Here's how the part is built. I have some questions about the finished solid (model axes, mm). A direction names the side the tool comes from. Coordinates: 2 decimals unless noted, no trailing zeros. Write each loop counter-clockwise with the first axis right and the second up, starting at its lowest first coordinate (ties: lowest second). Pieces come first, ordered by that corner, then holes.
Item 1: If I drill on line 1 (X direction, y = -0.5, z = 1.1); line 2 (Y direction, x = -34, z = 3.8); line 3 (X direction, y = -5.25, z = 1.55), over which ranges is the centre line in solid material (lowest first)?
Item 2: We'd pull the mould along X, two halves only. Please class faces 1 (the face through (1, 0, 0)), 2 (the face through (54.15, -0.27, 2.96)), 3 (the face through (-12.918, -2.873, 2.958)), 4 (the face through (15.819, 3.575, 2.958)): +X half, -X half, draft (parallel to the pull), parting line (faces both ways), or undercut.
Item 3: For faces 5 (the face through (-34.37, -5.53, 4.52)), 6 (the face through (-31, -10, 3)), 7 (the face through (-42.6, -7.3, 3)), which set-ups out of +Z, -Z, +X, -X, +Y, -Y let a thin tool reach every point of the face, with its end or its side?
Item 4: If we section it at A-A (x = 8.5): Please give me the cut outline in (y, z), then the cut area to 3 significant figures.
Item 5: If we section it at C-C (x = -6): Please give me the cut outline in (y, z).
Item 6: If we section it at B-B (z = 1.3): Count the separate pieces of the cut face and the enclosed holes in it, then the cut area to 3 significant figures.
Item 7: I'm going to push flat-ended pins straight in: pin 1 Ø1 at (y, z) = (8.5, 4) entering from -X; pin 2 Ø1.5 at (y, z) = (-8, 4.5) entering from -X; pin 3 Ø3 at (y, z) = (-6.5, 4.5) entering from +X. Where does each tip first touch, or does it pass through?
Item 8: If we section it at D-D (x = -29): Please give me the cut outline in (y, z), then the cut area to 3 significant figures.
from build123d import *

# Parameters (mm, degrees)
SKETCH1_R                                       = 4
SKETCH1_R_2                                     = 1.55
SKETCH1_R_3                                     = 7.5
BOSS_EXTRUDE1_DEPTH                             = 6
CSK_FOR_M5_FLAT_HEAD_MACHINE_SCREW1_D           = 5.5
CSK_FOR_M5_FLAT_HEAD_MACHINE_SCREW1_DEPTH       = 13.347633298
CSK_FOR_M5_FLAT_HEAD_MACHINE_SCREW1_CSINK_D     = 10.4
CSK_FOR_M5_FLAT_HEAD_MACHINE_SCREW1_CSINK_ANGLE = 90
CSK_FOR_M5_FLAT_HEAD_MACHINE_SCREW1_TIP         = 1.652366702
SKETCH7_R                                       = 1.55
CUT_EXTRUDE1_DEPTH                              = 3
SKETCH8_R                                       = 3
CUT_EXTRUDE2_DEPTH                              = 56.658073272


with BuildPart() as part:
    # Sketch1 → Boss-Extrude1 (new body)
    with BuildSketch(Plane.XY):
        with BuildLine():
            Line((-46.445530028, -10), (-15.598952553, -10))
            Line((-15.598952553, -10), (-13.098952553, -12.5))
            Line((-13.098952553, -12.5), (41.653218929, -12.5))
            ThreePointArc((41.653218929, -12.5), (54.153218929, 0), (41.653218929, 12.5))
            Line((41.653218929, 12.5), (-41.895881711, 12.5))
            ThreePointArc((-41.895881711, 12.5), (-50.825462961, 2.595635751), (-46.445530028, -10))
        make_face()
        with Locations((10.153527864, 0)):
            Circle(SKETCH1_R, mode=Mode.SUBTRACT)
        with Locations((15.103275332, 4.949747468)):
            Circle(SKETCH1_R_2, mode=Mode.SUBTRACT)
        with Locations(Location((5.203780395, 4.949747468, 0), (0, 0, 180))):
            Circle(SKETCH1_R_2, mode=Mode.SUBTRACT)
        with Locations(Location((15.103275332, -4.949747468, 0), (0, 0, 180))):
            Circle(SKETCH1_R_2, mode=Mode.SUBTRACT)
        with Locations((5.203780395, -4.949747468)):
            Circle(SKETCH1_R_2, mode=Mode.SUBTRACT)
        with Locations((-33.846472136, 0)):
            Circle(SKETCH1_R_2, mode=Mode.SUBTRACT)
        with Locations((-19.846472136, 0)):
            Circle(SKETCH1_R_3, mode=Mode.SUBTRACT)
        with Locations((-5.846472136, 0)):
            Circle(SKETCH1_R_2, mode=Mode.SUBTRACT)
    extrude(amount=BOSS_EXTRUDE1_DEPTH)

    # CSK for M5 Flat Head Machine Screw1
    with Locations(Plane.XY.offset(6)):
        with Locations((41.653218929, 0)):
            CounterSinkHole(CSK_FOR_M5_FLAT_HEAD_MACHINE_SCREW1_D / 2, CSK_FOR_M5_FLAT_HEAD_MACHINE_SCREW1_CSINK_D / 2, depth=CSK_FOR_M5_FLAT_HEAD_MACHINE_SCREW1_DEPTH, counter_sink_angle=CSK_FOR_M5_FLAT_HEAD_MACHINE_SCREW1_CSINK_ANGLE)
            with Locations((0, 0, -(CSK_FOR_M5_FLAT_HEAD_MACHINE_SCREW1_DEPTH + CSK_FOR_M5_FLAT_HEAD_MACHINE_SCREW1_TIP / 2))):  # 118° drill point
                Cone(0, CSK_FOR_M5_FLAT_HEAD_MACHINE_SCREW1_D / 2, CSK_FOR_M5_FLAT_HEAD_MACHINE_SCREW1_TIP, mode=Mode.SUBTRACT)

    # Sketch7 → Cut-Extrude1 (cut)
    with BuildSketch(Plane.XY.offset(6)):
        with Locations((-43.846472136, -6)):
            Circle(SKETCH7_R)
        with Locations((-35.846472136, -6)):
            Circle(SKETCH7_R)
    extrude(amount=-CUT_EXTRUDE1_DEPTH, mode=Mode.SUBTRACT)

    # Sketch8 → Cut-Extrude2 (cut, through all)
    with BuildSketch(Plane.XY.offset(3)):
        with Locations((-35.846472136, -6)):
            Circle(SKETCH8_R)
        with Locations((-43.846472136, -6)):
            Circle(SKETCH8_R)
    extrude(amount=-CUT_EXTRUDE2_DEPTH, mode=Mode.SUBTRACT)


solid = part.part
Answer list:
1. line 1: x = -51.08 to -35.31, -32.38 to -27.33, -12.36 to -7.31, -4.38 to 6.18, 14.12 to 38.95, 44.36 to 54.14
1. line 2: y = -10 to -1.54, 1.54 to 12.5
1. line 3: x = -49.99 to -46.75, -40.94 to -38.75, -32.94 to -25.2, -14.49 to 3.68, 6.72 to 13.58, 16.62 to 53
2. face 1: draft
2. face 2: +X half
2. face 3: undercut
2. face 4: undercut
3. face 5: +Z, -Z
3. face 6: +Z, -Z, -X, -Y
3. face 7: -Z
4. outline: (-12.5, 0) - (-3.64, 0) - (-3.64, 6) - (-12.5, 6) - close; (3.64, 0) - (12.5, 0) - (12.5, 6) - (3.64, 6) - close
4. area: 106 mm2
5. outline: (-12.5, 0) - (-1.54, 0) - (-1.54, 6) - (-12.5, 6) - close; (1.54, 0) - (12.5, 0) - (12.5, 6) - (1.54, 6) - close
6. separate pieces: 1
6. enclosed holes: 11
6. area: 2,070 mm2
7. pin 1: stops at x = -48.36
7. pin 2: stops at x = -48.9
7. pin 3: stops at x = 53.11
8. outline: (-10, 0) - (12.5, 0) - (12.5, 6) - (-10, 6) - close
8. area: 135 mm2
